from build123d import *

# Parameters (mm, degrees)
SKETCH3_W           = 2
SKETCH3_H           = 5
CUT_EXTRUDE6_DEPTH  = 25.176500961
BOSS_EXTRUDE4_DEPTH = 20
SKETCH2_R           = 3.3
CUT_EXTRUDE7_DEPTH  = 45.176500961


with BuildPart() as part:
    # Sketch1 → Revolve3 (revolve)
    with BuildSketch(Plane.XY):
        with BuildLine():
            Line((0, 0), (0, 6.982))
            Line((0, 6.982), (4.76, 6.982))
            Line((4.76, 6.982), (11.56, 7.937677676))
            Line((11.56, 7.937677676), (13.343138593, 6.154539083))
            ThreePointArc((13.343138593, 6.154539083), (13.880539746, 5.931940237), (14.4179409, 6.154539083))
            Line((14.4179409, 6.154539083), (16.96, 8.696598183))
            Line((16.96, 8.696598183), (22.676500961, 9.5))
            Line((22.676500961, 9.5), (22.676500961, 11.5))
            Line((22.676500961, 11.5), (24.176500961, 11.5))
            Line((24.176500961, 11.5), (24.176500961, 0))
            Line((24.176500961, 0), (0, 0))
        make_face()
    revolve(axis=Axis((24.176500961, 0, 0), (-1, 0, 0)))

    # Sketch3 → Cut-Extrude6 (cut, through all)
    with BuildSketch(Plane(origin=(24.176500961, 0, 0), x_dir=(0, 0, -1), z_dir=(1, 0, 0))):
        with Locations((-10.75, 0)):
            Rectangle(SKETCH3_W, SKETCH3_H)
        with Locations((10.75, 0)):
            Rectangle(SKETCH3_W, SKETCH3_H)
    extrude(amount=-CUT_EXTRUDE6_DEPTH, mode=Mode.SUBTRACT)

    # Sketch4 → Boss-Extrude4 (add)
    with BuildSketch(Plane(origin=(24.176500961, 0, 0), x_dir=(0, 0, -1), z_dir=(1, 0, 0))):
        with BuildLine():
            Line((-3, 4), (3, 4))
            ThreePointArc((3, 4), (0, -5), (-3, 4))
        make_face()
    extrude(amount=BOSS_EXTRUDE4_DEPTH)

    # Sketch2 → Cut-Extrude7 (cut, through all)
    with BuildSketch(Plane(origin=(0, 0, 0), x_dir=(0, 0, -1), z_dir=(1, 0, 0))):
        Circle(SKETCH2_R)
    extrude(amount=CUT_EXTRUDE7_DEPTH, mode=Mode.SUBTRACT)


solid = part.part
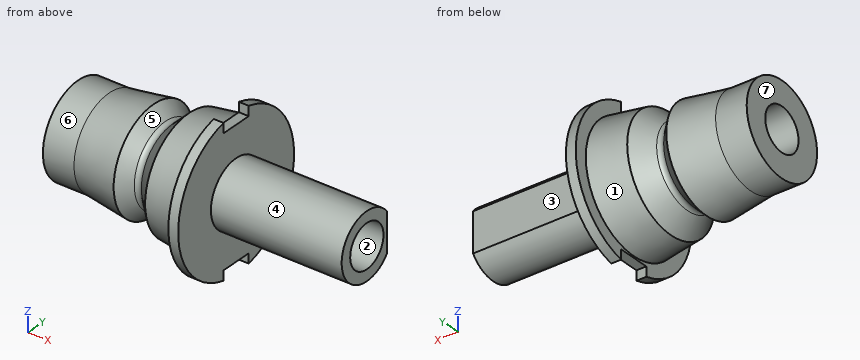
The model under review builds one solid part; all positions refer to its coordinate system, in mm. Face numbers are marked on the shaded views. A direction names the side the tool comes from. Give positions to 0.01 mm unless a question says otherwise; leave off trailing zeros. Write each loop counter-clockwise with the first axis right and the second up, starting at its lowest first coordinate (ties: lowest second). Pieces come first, ordered by that corner, then holes.
1. Add section D-D, the plane x = 15. Write out the cut boundary in (y, z), plus the area to 3 significant figures.
2. Tool access review of the marked faces 4, 5, 6 and 7: name each direction out of +Z, -Z, +X, -X, +Y, -Y from which nothing blocks a thin tool from reaching the whole face with its end or side.
3. Add section B-B, the plane z = 0. Write out the cut boundary in (x, y).
4. Add section C-C, the plane x = 34.5. Write out the cut boundary in (y, z).
5. Wall thickness on L1, parallel to Y at x = 35, z = 0; L2, parallel to Z at x = 29.5, y = 0; L3, parallel to Z at x = 23, y = 0: over which ranges is each line inside the solid? List them lowest first.
6. Draft analysis for pull direction Z (two halves, no side actions). For the marked faces 1, 2 and 3, state which applies: +Z half, -Z half, draft (parallel to the pull), parting line (faces both ways), or undercut.
7. For P1, Ø6, axis at x = 34.5, y = -2, coming from the +Z side; P2, Ø1.5, axis at x = 17, z = 0.5, coming from the +Y side; P3, Ø2, axis at y = -3, z = 5, coming from the +X side; P4, Ø6.5, axis at x = 31.5, z = 1, coming from the +Y side, all flat-tipped, find the tip position at first contact; note any pin that passes through.
8. Add section A-A, the plane y = 0. Write out the cut boundary in (x, z).
Worked answers:
1. outline: circle Ø13.47 at (0, 0); hole circle Ø6.6 at (0, 0)
1. area: 108 mm2
2. face 4: +X
2. face 5: none
2. face 6: -X
2. face 7: +Z, -Z, -X, +Y, -Y
3. outline: (0, -6.98) - (4.76, -6.98) - (11.56, -7.94) - (13.34, -6.15) arc R0.76 cw to (14.42, -6.15) - (16.96, -8.7) - (22.68, -9.5) - (22.68, -11.5) - (24.18, -11.5) - (24.18, -5) - (44.18, -5) - (44.18, -3.3) - (0, -3.3) - close; (0, 3.3) - (44.18, 3.3) - (44.18, 4) - (24.18, 4) - (24.18, 11.5) - (22.68, 11.5) - (22.68, 9.5) - (16.96, 8.7) - (14.42, 6.15) arc R0.76 cw to (13.34, 6.15) - (11.56, 7.94) - (4.76, 6.98) - (0, 6.98) - close
4. outline: (4, -3) - (4, 3) arc R5 ccw (long way) to start; hole circle Ø6.6 at (0, 0)
5. L1: y = -5 to -3.3, 3.3 to 4
5. L2: z = -5 to -3.3, 3.3 to 5
5. L3: z = -9.75 to -3.3, 3.3 to 9.75
6. face 1: parting line
6. face 2: undercut
6. face 3: draft
7. P1: stops at z = 5
7. P2: stops at y = 8.8
7. P3: stops at x = 44.18
7. P4: stops at y = 4
8. outline: (0, -6.98) - (4.76, -6.98) - (11.56, -7.94) - (13.34, -6.15) arc R0.76 cw to (14.42, -6.15) - (16.96, -8.7) - (22.68, -9.5) - (22.68, -9.75) - (24.18, -9.75) - (24.18, -5) - (44.18, -5) - (44.18, -3.3) - (0, -3.3) - close; (0, 3.3) - (44.18, 3.3) - (44.18, 5) - (24.18, 5) - (24.18, 9.75) - (22.68, 9.75) - (22.68, 9.5) - (16.96, 8.7) - (14.42, 6.15) arc R0.76 cw to (13.34, 6.15) - (11.56, 7.94) - (4.76, 6.98) - (0, 6.98) - close
